The listing builds one solid part. Answer for the finished solid, in the listing's coordinates (mm). A direction names the side the tool comes from. Give positions to 0.01 mm unless a question says otherwise; leave off trailing zeros. Loops run counter-clockwise (first coordinate to the right, second up) from the corner with the lowest first, then second, coordinate; pieces in that order, holes last. Notation, with made-up numbers: M 0.25,81.5 L 49.25,81.5 A15 cw 49.25,87.5 Z; hole C 64,-30.75 d4. An arc over 180 degrees is marked long. One line per item, written item: value. Start each with the question number.
Q1. Flat-ended cylindrical pins translate along their axes: pin 1 (1.5 mm diameter, centred on x = 54, y = 1, fed in from -Z); pin 2 (1.6 mm diameter, centred on x = 56, y = 4, fed in from +Z); pin 3 (3 mm diameter, centred on x = 30, z = 1.5, fed in from +Y) (3 decimals); pin 4 (0.9 mm diameter, centred on x = 57, y = 4.5, fed in from -Z). Find the tip coordinate at first contact, or state that the pin passes through.
Q2. A cutting plane is placed at A-A, the plane y = 0. State how many separate pieces and enclosed holes the cut face has, and give its area (3 significant figures).
Q3. Consider L1, parallel to X at y = 0, z = -3.75; L2, parallel to X at y = 0, z = -2.55; L3, parallel to Z at x = 6.5, y = 0 (3 decimals). Determine where each line is inside the solid, lowest interval first.
Q4. For faces 1 (the cylindrical face through (7, 3, 0)), 2 (the flat face through (58, 4, 1.588)), 3 (the flat face through (32, 3.175, 2)), determine the directions among +Z, -Z, +X, -X, +Y, -Y from which every point of the face is accessible in a straight line to the end or side of a thin tool.
Q5. A cutting plane is placed at C-C, the plane x = 25. Determine the outline of the cut face in (y, z) (3 decimals).
Q6. The mould has two halves that part along Z. Classify faces 4 (the flat face through (40, 0, -2)), 5 (the conical face through (74.78, 4.25, -0.17)), 6 (the cylindrical face through (43.913, -4.414, 0.035)): +Z half, -Z half, draft (parallel to the pull), parting line (faces both ways), or undercut.
from build123d import *

# Parameters (mm, degrees)
F0_R           = 6.125
F1_DEPTH       = 75
F2_R           = 3.175
F3_DEPTH       = 35
F4_R           = 3
F5_DEPTH       = 15
F6_SIZE2       = 3.4641016151
F6_SIZE        = 2
F8_DEPTH       = 6.126
F8_DEPTH_BACK  = 1.17
F10_DEPTH      = 6.1260001
F10_DEPTH_BACK = 6.1260001
F11_W          = 15
F11_H          = 3.175
F12_DEPTH      = 25.0000003725
F13_R          = 1.5
F14_DEPTH      = 4.9560001


with BuildPart() as f1:
    # F0 (on Right) → F1 (new body)
    with BuildSketch(Plane.YZ):
        Circle(F0_R)
    extrude(amount=F1_DEPTH)

    # F2 (on face) → F3 (cut)
    with BuildSketch(Plane.YZ.offset(75)):
        Circle(F2_R)
    extrude(amount=-F3_DEPTH, mode=Mode.SUBTRACT)

    # F4 (on face) → F5 (cut)
    with BuildSketch(Plane(origin=(0, 0, 0), x_dir=(0, -1, 0), z_dir=(-1, 0, 0))):
        Circle(F4_R)
    extrude(amount=-F5_DEPTH, mode=Mode.SUBTRACT)

    # F6
    f6_edges = [f1.edges().sort_by_distance(p)[0] for p in [
        (75, -6.125, 0),
    ]]
    f6_side = f1.faces().sort_by_distance((75, -5.951759, 0))[0]
    chamfer(f6_edges, length=F6_SIZE, length2=F6_SIZE2, reference=f6_side)

    # F7 (on Top) → F8 (cut, two sides)
    with BuildSketch(Plane.XY) as f8_sk:
        with BuildLine():
            Line((44, 3.175), (20, 3.175))
            ThreePointArc((20, 3.175), (16.825, 0), (20, -3.175))
            Line((20, -3.175), (44, -3.175))
            ThreePointArc((44, -3.175), (47.175, 0), (44, 3.175))
        make_face()
    extrude(amount=F8_DEPTH, mode=Mode.SUBTRACT)
    extrude(f8_sk.sketch, amount=-F8_DEPTH_BACK, mode=Mode.SUBTRACT)

    # F9 (on Front) → F10 (cut, two sides)
    with BuildSketch(Plane.XZ) as f10_sk:
        with BuildLine():
            Line((70, 1.5875), (45.5, 1.5875))
            ThreePointArc((45.5, 1.5875), (43.9125, 0), (45.5, -1.5875))
            Line((45.5, -1.5875), (70, -1.5875))
            ThreePointArc((70, -1.5875), (71.5875, 0), (70, 1.5875))
        make_face()
    extrude(amount=-F10_DEPTH, mode=Mode.SUBTRACT)
    extrude(f10_sk.sketch, amount=F10_DEPTH_BACK, mode=Mode.SUBTRACT)

    # F11 (on Front) → F12 (cut)
    with BuildSketch(Plane.XZ):
        with Locations((70.5, 0)):
            Rectangle(F11_W, F11_H)
    extrude(amount=F12_DEPTH, mode=Mode.SUBTRACT)

    # F13 (on face) → F14 (cut, through all)
    with BuildSketch(Plane.XY.offset(-1.17)):
        with Locations((25, 0)):
            Circle(F13_R)
        with Locations((30, 0)):
            Circle(F13_R)
        with Locations((35, 0)):
            Circle(F13_R)
    extrude(amount=-F14_DEPTH, mode=Mode.SUBTRACT)


solid = f1.part
Answer block:
1. pin 1: z = -6.12
1. pin 2: z = 5.22
1. pin 3: y = 6.125
1. pin 4: z = -4.59
2. separate pieces: 5
2. enclosed holes: 0
2. area: 365 mm^2
3. L1: 0 to 23.5, 26.5 to 28.5, 31.5 to 33.5, 36.5 to 75
3. L2: 15 to 23.5, 26.5 to 28.5, 31.5 to 33.5, 36.5 to 40
3. L3: -6.125 to -3, 3 to 6.125
4. face 1: -X
4. face 2: +Y, -Y
4. face 3: +Z
5. outline: M -3.175,-1.17 L -3.175,5.238 A6.125 ccw -1.5,-5.938 L -1.5,-1.17 Z; M 1.5,-5.938 A6.125 ccw 3.175,5.238 L 3.175,-1.17 L 1.5,-1.17 Z
6. face 4: draft
6. face 5: parting line
6. face 6: undercut
